The drawing under review shows one solid part. Ordinate dimensions are in mm from its lowest x, y, z. A direction names the side the tool comes from. Give positions to 0.01 mm unless a question says otherwise; leave off trailing zeros. Write each loop counter-clockwise with the first axis right and the second up, starting at its lowest first coordinate (ties: lowest second). Pieces come first, ordered by that corner, then holes. Notation, with made-up numbers: (13, 87.5) - (32, 87.5) arc R34 ccw to (32, 119.5) - close; hole circle Ø3 at (83.25, 55.5). An arc over 180 degrees is marked (long way). Write item = value, one per line.
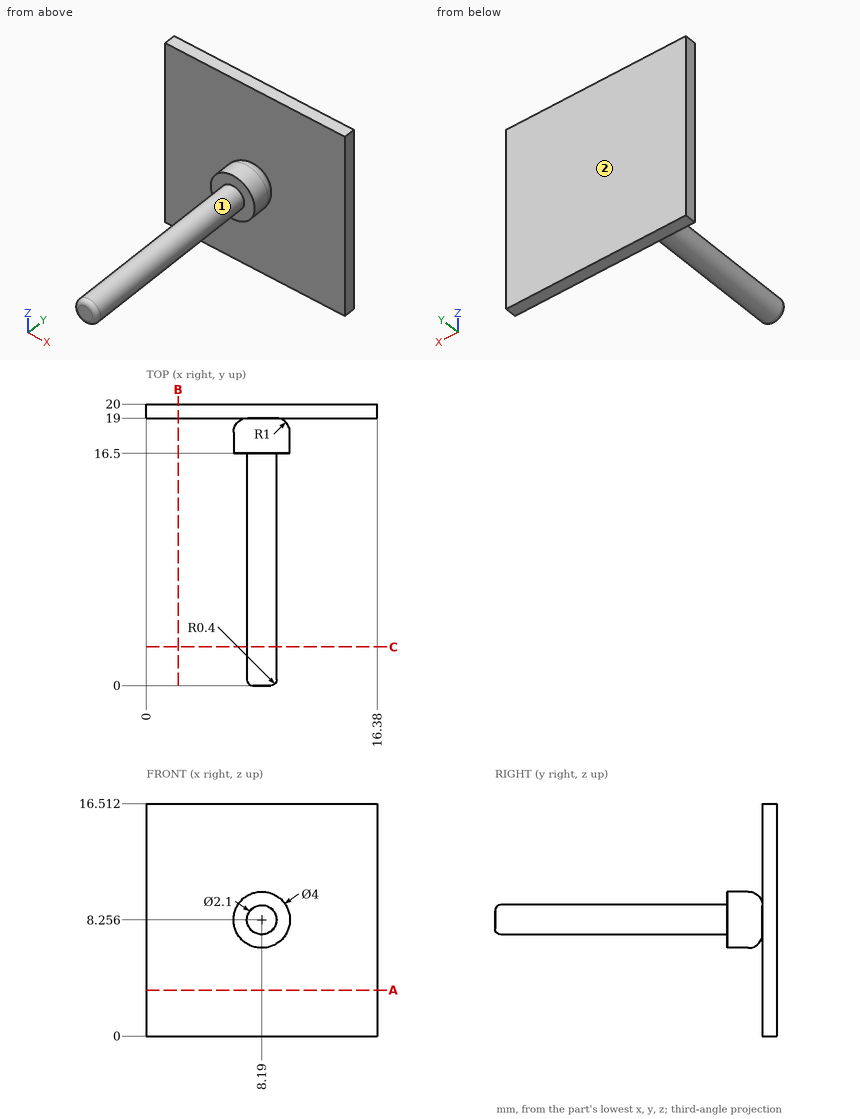
1. Take a section at C-C on y = 2.75. Give the boundary of the cut face in (x, z).
Findings below:
outline = circle Ø2.1 at (8.19, 8.26)
2. Take a section at A-A on z = 3.25. Give the boundary of the cut face in (x, y), and give its area (3 significant figures).
Findings below:
outline = (0, 19) - (16.38, 19) - (16.38, 20) - (0, 20) - close
area = 16.4 mm²
3. Insertion check: P1, Ø2, axis at y = 3.5, z = 9.5, coming from the -X side; P2, Ø3, axis at x = 6, z = 2.5, coming from the -Y side. Each pin has a flat end and moves straight along its axis. Give the tip position at first contact, or say it passes through.
Findings below:
P1 = 7.17
P2 = 19
4. For line 1 (Y direction, x = 4.5, z = 2.5); line 2 (Z direction, x = 8.25, y = 11.75) (1 decimal); line 3 (Y direction, x = 6.5, z = 8.25) (1 decimal), list the stretches that pass through material, from the lowest coordinate up. Write a range as from..to.
Findings below:
line_1 = 19..20
line_2 = 7.2..9.3
line_3 = 16.5..18.7, 19..20
5. Take a section at B-B on x = 2.25. Give the boundary of the cut face in (y, z).
Findings below:
outline = (19, 0) - (20, 0) - (20, 16.51) - (19, 16.51) - close
6. Machinability: for the marked faces 1 and 2, which of the approach directions +Z, -Z, +X, -X, +Y, -Y give a long, thin tool a straight path to every point of the face, cutting with its end or side? Answer none if there is none.
Findings below:
face_1 = -Y
face_2 = +Z, -Z, +X, -X, +Y
